```python
from build123d import *

# Parameters (mm, degrees)
SKETCH1_W           = 30
SKETCH1_H           = 60
SKETCH1_W_2         = 27.6
SKETCH1_H_2         = 57.6
BOSS_EXTRUDE1_DEPTH = 1955
SKETCH4_R           = 3.5
CUT_EXTRUDE3_DEPTH  = 1957.150556578
SKETCH5_R           = 4.25
CUT_EXTRUDE4_DEPTH  = 1957.150556578


with BuildPart() as part:
    # Sketch1 → Boss-Extrude1 (new body)
    with BuildSketch(Plane.XY):
        with Locations((15, 30)):
            Rectangle(SKETCH1_W, SKETCH1_H)
        with Locations((15, 30)):
            Rectangle(SKETCH1_W_2, SKETCH1_H_2, mode=Mode.SUBTRACT)
    extrude(amount=BOSS_EXTRUDE1_DEPTH)

    # Sketch4 → Cut-Extrude3 (cut, through all)
    with BuildSketch(Plane(origin=(30, 0, 0), x_dir=(0, 0, -1), z_dir=(1, 0, 0))):
        with Locations((-1452.5, 40)):
            Circle(SKETCH4_R)
        with Locations((-1452.5, 20)):
            Circle(SKETCH4_R)
        with Locations((-502.5, 40)):
            Circle(SKETCH4_R)
        with Locations((-502.5, 20)):
            Circle(SKETCH4_R)
    extrude(amount=-CUT_EXTRUDE3_DEPTH, mode=Mode.SUBTRACT)

    # Sketch5 → Cut-Extrude4 (cut, through all)
    with BuildSketch(Plane(origin=(30, 0, 0), x_dir=(0, 0, -1), z_dir=(1, 0, 0))):
        with Locations((-15, 15)):
            Circle(SKETCH5_R)
        with Locations((-65, 45)):
            Circle(SKETCH5_R)
        with Locations((-1890, 45)):
            Circle(SKETCH5_R)
        with Locations((-1940, 15)):
            Circle(SKETCH5_R)
    extrude(amount=-CUT_EXTRUDE4_DEPTH, mode=Mode.SUBTRACT)


solid = part.part
```
Check sheet for the modelled part. Datum: model origin and axes. Units: mm. Coordinates: 2 decimals unless noted, no trailing zeros. Loops run counter-clockwise (first coordinate to the right, second up) from the corner with the lowest first, then second, coordinate; pieces in that order, holes last.
1) Sectioned sample at B-B (x = 8.25). Record the boundary of the cut face in (y, z).
2) Sectioned sample at A-A (z = 1640). Record the boundary of the cut face in (x, y), and give its area (3 significant figures).
3) Material ranges on probe 1 along Y at (x, z) = (29.7, 1452.5); probe 2 along Y at (x, z) = (27.5, 1376.5); probe 3 along X at (y, z) = (34.5, 1143), recorded low to high.
4) Release check for a two-part mould opening along X. For faces 1 (the face through (0.5, 39, 1955)), 2 (the face through (30, 30, 964)), 3 (the face through (1.2, 30, 964)), 4 (the face through (28.8, 30, 964)) record: released by +X, released by -X, zero draft, split by the parting line, or undercut.
Check sheet entries:
1. outline: (0, 0) - (1.2, 0) - (1.2, 1955) - (0, 1955) - close; (58.8, 0) - (60, 0) - (60, 1955) - (58.8, 1955) - close
2. outline: (0, 0) - (30, 0) - (30, 60) - (0, 60) - close; hole (1.2, 1.2) - (28.8, 1.2) - (28.8, 58.8) - (1.2, 58.8) - close
2. area: 210 mm2
3. probe 1: y = 0 to 16.5, 23.5 to 36.5, 43.5 to 60
3. probe 2: y = 0 to 1.2, 58.8 to 60
3. probe 3: x = 0 to 1.2, 28.8 to 30
4. face 1: zero draft
4. face 2: released by +X
4. face 3: undercut
4. face 4: undercut
